Can you work these out from the model? Positions are in its coordinate system, mm. A direction names the side the tool comes from. Give positions to 0.01 mm unless a question says otherwise; leave off trailing zeros. Loops run counter-clockwise (first coordinate to the right, second up) from the corner with the lowest first, then second, coordinate; pieces in that order, holes last. Notation, with made-up numbers: (-11, 29) -> (10, 29) arc R21 cw to (10, 38) -> close; hole circle Ø2 at (46.5, -33). An arc over 180 degrees is marked (long way). Return JSON: item names as keys, results as strings. Group by question number.
Q1. Suppose I cut it at B-B, the plane y = 76. Please give me the cut outline in (x, z).
Q2. Suppose I cut it at A-A, the plane z = 1. Please give me the cut outline in (x, y).
Q3. Thinking about a two-plate mould opening in Z: for faces 1 (the flat face through (36, 41, 0)), 2 (the flat face through (-1, 41, -25)), 3 (the flat face through (1, 41, 25)), 4 (the cylindrical face through (35, 56, 20)), which applies, pulls with the +Z half, pulls with the -Z half, needs draft (parallel to the pull), parting line crosses it, or undercut?
Q4. Which directions (+Z, -Z, +X, -X, +Y, -Y) give clear straight access to the entire face, cutting with the end or side of a thin tool? Please do faces 5 (the cylindrical face through (35, 56, -20)), 6 (the flat face through (34.5, 43, 0)), 7 (the flat face through (35, 82.5, 0)).
Q5. I need wall thicknesses on line 1 along Z through (x, y) = (11.5, 44.5); line 2 along X through (y, z) = (48, 13); line 3 along Y through (x, z) = (-2, -19.5). Which ranges of each line are inside material? Lowest first, please. Write a range as [from, to].
Q6. Suppose I cut it at C-C, the plane x = 27.5. Please give me the cut outline in (y, z), and give its area (3 significant figures).
Q7. Suppose I cut it at D-D, the plane y = 55.5. Please give me the cut outline in (x, z), and give its area (3 significant figures).
Q8. Will this pin go through, and if not, where does the flat tip stop? pin 1 (14 mm diameter, centred on x = 7.5, z = 7, fed in from +Y).
Autodesk Inventor part; units mm, degrees
ref_plane "YZ Plane" through (0, 0, 0) normal (1, 0, 0) x (0, 1, 0)
ref_plane "XZ Plane" through (0, 0, 0) normal (0, 1, 0) x (-1, 0, 0)
ref_plane "XY Plane" through (0, 0, 0) normal (0, 0, 1) x (1, 0, 0)
sketch "Boceto3" plane through (0, 0, 0) normal (0, 1, 0) x (-1, 0, 0)
  line L0 (36, -25) -> (-36, -25)
  line L1 (-36, -25) -> (-36, 25)
  line L2 (-36, 25) -> (36, 25)
  line L3 (36, 25) -> (36, -25)
  point P0 (0, 0)
  point P1 (36, 0)
  point P2 (0, -25)
  dimension "d8" = 72
  dimension "d9" = 50
extrude "Extrusión2" add sketch "Boceto3" along normal blind 82.5
sketch "Boceto5" plane through (0, 82.5, 0) normal (0, 1, 0) x (1, 0, 0)
  line L0 (-34.5, -23.5) -> (34.5, -23.5)
  line L1 (34.5, -23.5) -> (34.5, 23.5)
  line L2 (34.5, 23.5) -> (-34.5, 23.5)
  line L3 (-34.5, 23.5) -> (-34.5, -23.5)
  line L4 (-36, 25) -> (-36, -25)
  line L5 (36, 25) -> (-36, 25)
  line L6 (36, -25) -> (36, 25)
  line L7 (-36, -25) -> (36, -25)
  point P0 (0, 0)
  dimension "d12" = 1.5
  dimension "d13" = 1.5
  dimension "d14" = 1.5
  dimension "d15" = 1.5
extrude "Extrusión3" cut sketch "Boceto5" against normal blind 81 contours L3 L2 L1 L0
sketch "Boceto6" plane through (36, 0, 25) normal (1, 0, 0) x (0, 0, -1)
  line L0 (10, 61) -> (40, 61)
  line L1 (45, 56) -> (45, 56)
  line L2 (40, 51) -> (10, 51)
  line L3 (5, 56) -> (5, 56)
  line L4 (0, 82.5) -> (50, 82.5)
  arc A0 (10, 61) -> (5, 56) centre (10, 56) ccw
  arc A1 (5, 56) -> (10, 51) centre (10, 56) ccw
  arc A2 (45, 56) -> (40, 61) centre (40, 56) ccw
  arc A3 (40, 51) -> (45, 56) centre (40, 56) ccw
  point P0 (25, 0)
  point P1 (5, 61)
  point P2 (45, 51)
  point P3 (5, 51)
  point P4 (25, 61)
  point P5 (25, 82.5)
  dimension "d18" = 21.5
  dimension "d19" = 40
  dimension "d20" = 10
  dimension "d21" = 5
extrude "Extrusión4" cut sketch "Boceto6" against normal through all
properties part number "Caja2_ConOrificios"
Ans:
{
 "1": {"outline": "(-36, -25) -> (36, -25) -> (36, 25) -> (-36, 25) -> close; hole (-34.5, -23.5) -> (34.5, -23.5) -> (34.5, 23.5) -> (-34.5, 23.5) -> close"},
 "2": {"outline": "(-36, 0) -> (36, 0) -> (36, 51) -> (34.5, 51) -> (34.5, 1.5) -> (-34.5, 1.5) -> (-34.5, 51) -> (-36, 51) -> close; (-36, 61) -> (-34.5, 61) -> (-34.5, 82.5) -> (-36, 82.5) -> close; (34.5, 61) -> (36, 61) -> (36, 82.5) -> (34.5, 82.5) -> close"},
 "3": {"face 1": "needs draft", "face 2": "pulls with the -Z half", "face 3": "pulls with the +Z half", "face 4": "undercut"},
 "4": {"face 5": "+X, -X", "face 6": "+Y", "face 7": "+Z, -Z, +X, -X, +Y"},
 "5": {"line 1": "z = [-25, -23.5], [23.5, 25]", "line 2": "x = [-36, -34.5], [34.5, 36]", "line 3": "y = [0, 1.5]"},
 "6": {"outline": "(0, -25) -> (82.5, -25) -> (82.5, -23.5) -> (1.5, -23.5) -> (1.5, 23.5) -> (82.5, 23.5) -> (82.5, 25) -> (0, 25) -> close", "area": "318 mm^2"},
 "7": {"outline": "(-36, -25) -> (36, -25) -> (36, -19.97) -> (34.5, -19.97) -> (34.5, -23.5) -> (-34.5, -23.5) -> (-34.5, -19.97) -> (-36, -19.97) -> close; (-36, 19.97) -> (-34.5, 19.97) -> (-34.5, 23.5) -> (34.5, 23.5) -> (34.5, 19.97) -> (36, 19.97) -> (36, 25) -> (-36, 25) -> close", "area": "237 mm^2"},
 "8": {"pin 1": "stops at y = 1.5"}
}
